Job drawing, mm, ordinate dimensions from the low corner. One solid piece. Give positions to 0.01 mm unless a question says otherwise; leave off trailing zeros. Loops run counter-clockwise (first coordinate to the right, second up) from the corner with the lowest first, then second, coordinate; pieces in that order, holes last.
Item 1: Probe probe 1 along Y at (x, z) = (38.1, 0.9); probe 2 along X at (y, z) = (61.5, 1.4); probe 3 along Y at (x, z) = (63.5, 2.15). List the from-to ranges inside material, lowest first.
Item 2: Saw through at C-C on x = 12.7. Give the cut face in (y, z) (1 decimal), plus the area to 3 significant figures.
Item 3: Drop flat-ended pins along their axis: P1, Ø4.5, axis at x = 12.7, y = 63.5, coming from the -Z side; P2, Ø1, axis at x = 68, z = 1, coming from the -Y side; P3, Ø1, axis at y = 24.5, z = 1.5, coming from the -X side. Give the stop position or say it passes through.
Item 4: Saw through at A-A on x = 38.1. Give the cut face in (y, z) (1 decimal).
Item 5: Saw through at D-D on z = 1.5. Give the cut face in (x, y).
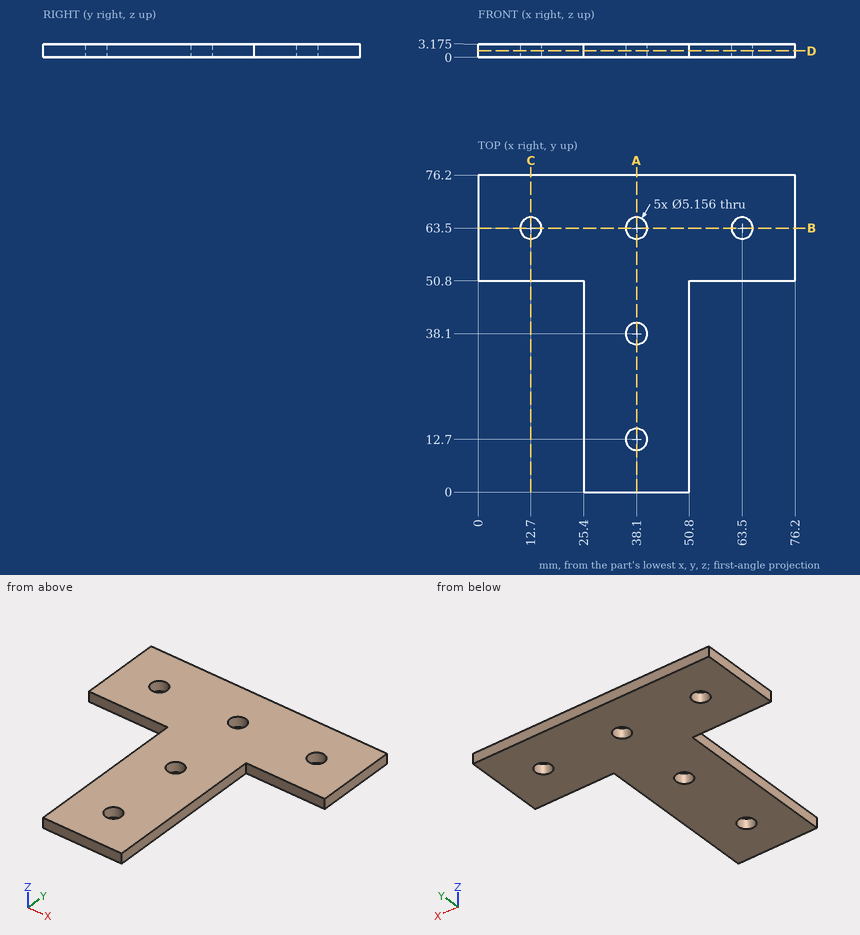
Results below:
1. probe 1: y = 0 to 10.12, 15.28 to 35.52, 40.68 to 60.92, 66.08 to 76.2
1. probe 2: x = 0 to 11.07, 14.33 to 36.47, 39.73 to 61.87, 65.13 to 76.2
1. probe 3: y = 50.8 to 60.92, 66.08 to 76.2
2. outline: (50.8, 0) - (60.9, 0) - (60.9, 3.2) - (50.8, 3.2) - close; (66.1, 0) - (76.2, 0) - (76.2, 3.2) - (66.1, 3.2) - close
2. area: 64.3 mm2
3. P1: passes through
3. P2: stops at y = 50.8
3. P3: stops at x = 25.4
4. outline: (0, 0) - (10.1, 0) - (10.1, 3.2) - (0, 3.2) - close; (15.3, 0) - (35.5, 0) - (35.5, 3.2) - (15.3, 3.2) - close; (40.7, 0) - (60.9, 0) - (60.9, 3.2) - (40.7, 3.2) - close; (66.1, 0) - (76.2, 0) - (76.2, 3.2) - (66.1, 3.2) - close
5. outline: (0, 50.8) - (25.4, 50.8) - (25.4, 0) - (50.8, 0) - (50.8, 50.8) - (76.2, 50.8) - (76.2, 76.2) - (0, 76.2) - close; hole circle Ø5.16 at (12.7, 63.5); hole circle Ø5.16 at (38.1, 12.7); hole circle Ø5.16 at (38.1, 38.1); hole circle Ø5.16 at (38.1, 63.5); hole circle Ø5.16 at (63.5, 63.5)
